The listing builds one solid part. Answer for the finished solid, in the listing's coordinates (mm). A direction names the side the tool comes from. Round coordinates to 2 decimals unless told otherwise and drop trailing zeros. Order: outer loops, then holes, each group sorted by start corner. A loop starts at its lowest first (then second) coordinate and runs counter-clockwise, first axis right, second up. Notation, with made-up numbers: (25.5, 28) - (48.5, 28) arc R25 cw to (48.5, 47) - close; hole circle Ø9 at (-22.5, -32.5). An arc over 180 degrees is marked (long way). Use CSV: the item, a comma, the result in double quotes. Start each with the question number.
Item 1: Flat-ended cylindrical pins translate along their axes: P1, Ø4, axis at y = -159, z = -8, coming from the +X side; P2, Ø2, axis at x = 5.5, y = -11, coming from the -Z side; P3, Ø9.5, axis at x = 1.5, y = -69.5, coming from the -Z side; P4, Ø9.5, axis at y = -108, z = 3, coming from the -X side. Find the tip coordinate at first contact, or state that the pin passes through.
Item 2: Straight lines are drawn through the part: line 1 along Y through (x, z) = (12, -1.5); line 2 along Y through (x, z) = (4.5, 8.5); line 3 along Y through (x, z) = (2, 6.5). For each, find the intervals that lie inside material, in ascending order. Write a range as [from, to].
Item 3: Find section C-C, the plane y = -90. Give the vertices of the cut face in (x, z).
Item 4: Determine the mould class of faces 4 (the flat face through (0, 200, 0)), 5 (the flat face through (0, -113, 11.6)), 6 (the flat face through (0, -200, 0)) for opening direction Y: +Y half, -Y half, draft (parallel to the pull), parting line (faces both ways), or undercut.
Item 5: Find section A-A, the plane z = -4. Give the vertices of the cut face in (x, y), plus the area to 3 significant figures.
Item 6: Find section B-B, the plane y = -165. Give the vertices of the cut face in (x, z), plus the area to 3 significant figures.
Item 7: For faces 1 (the flat face through (0, -100, 6)), 2 (the flat face through (0, -66, 11.6)), 3 (the cylindrical face through (-1.953, -2.8, 14.872)), determine the directions among +Z, -Z, +X, -X, +Y, -Y from which every point of the face is accessible in a straight line to the end or side of a thin tool.
```python
from build123d import *

# Parameters (mm, degrees)
F0_R     = 15
F1_DEPTH = 200
F2_R     = 10
F3_DEPTH = 200
F4_R     = 10
F5_DEPTH = 200
F6_W     = 24.5755761862
F6_H     = 72.3862349987
F7_DEPTH = 58.4
F8_DEPTH = 11.6


with BuildPart() as f1:
    # F0 (on Front) → F1 (new body, symmetric)
    with BuildSketch(Plane.XZ):
        Circle(F0_R)
    extrude(amount=F1_DEPTH, both=True)

    # F2 (on Right) → F3 (cut, symmetric)
    with BuildSketch(Plane.YZ):
        with Locations((188, 0)):
            Circle(F2_R)
        with Locations((-188, 0)):
            Circle(F2_R)
    extrude(amount=F3_DEPTH, both=True, mode=Mode.SUBTRACT)

    # F4 (on Right) → F5 (cut, symmetric)
    with BuildSketch(Plane.YZ):
        with Locations((-90, 0)):
            Circle(F4_R)
    extrude(amount=F5_DEPTH, both=True, mode=Mode.SUBTRACT)

    # F6 (on Top) → F7 (cut)
    with BuildSketch(Plane.XY):
        with Locations((0, -89.3657207489)):
            Rectangle(F6_W, F6_H)
    extrude(amount=-F7_DEPTH, mode=Mode.SUBTRACT)

    # F8 (cut): faces of the model
    f8_faces = [f1.faces().sort_by_distance(p)[0] for p in [
        (0, -66.5863016248, 0),
        (0, -112.7794191241, 0),
    ]]
    extrude(f8_faces, amount=-F8_DEPTH, mode=Mode.SUBTRACT)


solid = f1.part
```
Worked out:
1,P1,"stops at x = 13.75"
1,P2,"stops at z = -14.31"
1,P3,"stops at z = 11.6"
1,P4,"stops at x = -15"
2,line 1,"y = [-200, -197.89], [-178.11, -125.56], [-53.17, 178.11], [197.89, 200]"
2,line 2,"y = [-200, -193.27], [-182.73, -125.56], [-100, -95.27], [-84.73, -80], [-53.17, 182.73], [193.27, 200]"
2,line 3,"y = [-200, -195.6], [-180.4, -125.56], [-100, -97.6], [-82.4, -80], [-53.17, 180.4], [195.6, 200]"
3,outline,"(-11.18, 10) - (11.18, 10) arc R15 ccw to start"
4,face 4,"+Y half"
4,face 5,"undercut"
4,face 6,"-Y half"
5,outline,"(-14.46, -200) - (14.46, -200) - (14.46, -197.17) - (-14.46, -197.17) - close; (-14.46, -178.83) - (14.46, -178.83) - (14.46, -99.17) - (12.29, -99.17) - (12.29, -125.56) - (-12.29, -125.56) - (-12.29, -99.17) - (-14.46, -99.17) - close; (-14.46, -80.83) - (-12.29, -80.83) - (-12.29, -53.17) - (12.29, -53.17) - (12.29, -80.83) - (14.46, -80.83) - (14.46, 178.83) - (-14.46, 178.83) - close; (-14.46, 197.17) - (14.46, 197.17) - (14.46, 200) - (-14.46, 200) - close"
5,area,"8,650 mm²"
6,outline,"circle Ø30 at (0, 0)"
6,area,"707 mm²"
7,face 1,"-Z"
7,face 2,"-Z, +X, -X"
7,face 3,"+Y, -Y"
